The listing builds one solid part. Answer for the finished solid, in the listing's coordinates (mm). A direction names the side the tool comes from. Round coordinates to 2 decimals unless told otherwise and drop trailing zeros. Loops run counter-clockwise (first coordinate to the right, second up) from the corner with the lowest first, then second, coordinate; pieces in that order, holes last. Notation, with made-up numbers: (84.25, 29) - (88.25, 29) arc R22 cw to (88.25, 61) - close; hole circle Ø8 at (13, -6.5). An arc over 180 degrees is marked (long way). Write item = value, one per line. Start each with the question number.
1) Section B-B, the plane z = -0.95 is taken. Determine the outline of the cut face in (x, y).
2) A tool of negligible diameter and unlimited length cuts with its end or side. For faces 1 (the flat face through (20, 81, -2)), 2 (the flat face through (-10, 76, -2)), 3 (the flat face through (-20, 81, -2)), from which of +Z, -Z, +X, -X, +Y, -Y can it reach the whole face along a straight path? Write none if from no direction.
3) Section C-C, the plane y = 24 is taken. Determine the outline of the cut face in (x, z), and give its area (3 significant figures).
4) Given pin 1 Ø3 at (x, z) = (-12.5, -2.5) entering from +Y; pin 2 Ø1.5 at (y, z) = (93.5, -2.5) entering from +X; pin 3 Ø1.5 at (y, z) = (151, -4.5) entering from -X, each flat-ended and moving along its own axis, determine where each tip first touches the part or whether it passes through.
5) Section D-D, the plane x = 0 is taken. Determine the outline of the cut face in (y, z).
6) Straight lines are drawn through the part: line 1 along X through (y, z) = (-21, -3.45); line 2 along Y through (x, z) = (0, -3.6); line 3 along X through (y, z) = (89, -4.15). For each, find the intervals that lie inside material, in ascending order.
7) Section A-A, the plane y = -21 is taken. Determine the outline of the cut face in (x, z).
8) For a pull along X with two mould halves and no side action, classify faces 4 (the cylindrical face through (0, 165, -3)), 5 (the flat face through (-59.44, -8.38, -2.46)), 6 (the cylindrical face through (0, 180, -2)), 7 (the flat face through (100, -21, -2)) as released by +X, released by -X, zero draft, split by the parting line, or undercut.
Autodesk Inventor part; units mm, degrees
ref_plane "YZ Plane" through (0, 0, 0) normal (1, 0, 0) x (0, 1, 0)
ref_plane "XZ Plane" through (0, 0, 0) normal (0, 1, 0) x (-1, 0, 0)
ref_plane "XY Plane" through (0, 0, 0) normal (0, 0, 1) x (1, 0, 0)
sketch "Sketch1" plane through (0, 0, 0) normal (0, 0, 1) x (1, 0, 0)
  line L0 (0, 0) -> (0, 91.5348) construction
  line L1 (-93.5855, 0) -> (93.5855, 0) construction
  arc A0 (20, 160) -> (-20, 160) centre (0, 160) ccw
  line L2 (-20, 160) -> (-20, 0)
  line L3 (-20, 0) -> (-100, -17)
  line L4 (-100, -17) -> (-100, -25)
  line L5 (-100, -25) -> (100, -25)
  line L6 (100, -25) -> (100, -17)
  line L7 (20, 160) -> (20, 0)
  line L8 (20, 0) -> (100, -17)
  dimension "d0" = 20
  dimension "d1" = 185
  dimension "d2" = 8
  dimension "d3" = 25
  dimension "d4" = 200
extrude "Extrusion1" add sketch "Sketch1" against normal blind 5
sketch "Sketch2" plane through (0, 0, 0) normal (0, 0, 1) x (1, 0, 0)
  line L0 (0, 20) -> (0, 130) construction
  line L1 (10, 20) -> (10, 130)
  line L2 (-10, 130) -> (-10, 20)
  arc A0 (-10, 20) -> (10, 20) centre (0, 20) ccw
  arc A1 (10, 130) -> (-10, 130) centre (0, 130) ccw
  arc A2 (20, 160) -> (-20, 160) centre (0, 160) ccw
  point P0 (0, 0)
  point P1 (0, 75)
  point P2 (0, 10)
  dimension "d7" = 30
  dimension "d8" = 10
  dimension "d9" = 110
extrude "Extrusion2" cut sketch "Sketch2" against normal up to surface (5 mm away)
sketch "Sketch3" plane through (0, 0, 0) normal (0, 0, 1) x (1, 0, 0)
  line L0 (-100, -25) -> (100, -25)
  point P0 (0, 0)
  point P1 (-90, -21)
  point P2 (-45, -21)
  point P3 (0, -21)
  point P4 (45, -21)
  point P5 (90, -21)
  dimension "d12" = 45
  dimension "d13" = 45
  dimension "d14" = 45
  dimension "d15" = 45
  dimension "d16" = 4
hole "Hole1" at (-90, -21, 0) at (-45, -21, 0) at (0, -21, 0) at (45, -21, 0) at (90, -21, 0) direction (0, 0, -1) diameter 5 depth 5
sketch "Sketch4" plane through (0, 0, 0) normal (0, 0, 1) x (1, 0, 0)
  arc A0 (20, 160) -> (-20, 160) centre (0, 160) ccw
  point P0 (0, 0)
hole "Hole2" at (0, 160, 0) direction (0, 0, -1) diameter 10 depth 5
properties part number "03A"
Geometry check:
q1.outline = (-100, -25) - (100, -25) - (100, -17) - (20, 0) - (20, 160) arc R20 ccw to (-20, 160) - (-20, 0) - (-100, -17) - close; hole circle Ø5 at (-90, -21); hole circle Ø5 at (-45, -21); hole (-10, 20) arc R10 ccw to (10, 20) - (10, 130) arc R10 ccw to (-10, 130) - close; hole circle Ø10 at (0, 160); hole circle Ø5 at (0, -21); hole circle Ø5 at (45, -21); hole circle Ø5 at (90, -21)
q2.face_1 = +Z, -Z, +X, +Y
q2.face_2 = +Z, -Z
q2.face_3 = +Z, -Z, -X, +Y
q3.outline = (-20, -5) - (-10, -5) - (-10, 0) - (-20, 0) - close; (10, -5) - (20, -5) - (20, 0) - (10, 0) - close
q3.area = 100 mm2
q4.pin_1 = 176.7
q4.pin_2 = 20
q4.pin_3 = -20
q5.outline = (-25, -5) - (-23.5, -5) - (-23.5, 0) - (-25, 0) - close; (-18.5, -5) - (10, -5) - (10, 0) - (-18.5, 0) - close; (140, -5) - (155, -5) - (155, 0) - (140, 0) - close; (165, -5) - (180, -5) - (180, 0) - (165, 0) - close
q6.line_1 = -100 to -92.5, -87.5 to -47.5, -42.5 to -2.5, 2.5 to 42.5, 47.5 to 87.5, 92.5 to 100
q6.line_2 = -25 to -23.5, -18.5 to 10, 140 to 155, 165 to 180
q6.line_3 = -20 to -10, 10 to 20
q7.outline = (-100, -5) - (-92.5, -5) - (-92.5, 0) - (-100, 0) - close; (-87.5, -5) - (-47.5, -5) - (-47.5, 0) - (-87.5, 0) - close; (-42.5, -5) - (-2.5, -5) - (-2.5, 0) - (-42.5, 0) - close; (2.5, -5) - (42.5, -5) - (42.5, 0) - (2.5, 0) - close; (47.5, -5) - (87.5, -5) - (87.5, 0) - (47.5, 0) - close; (92.5, -5) - (100, -5) - (100, 0) - (92.5, 0) - close
q8.face_4 = undercut
q8.face_5 = released by -X
q8.face_6 = split by the parting line
q8.face_7 = released by +X
